```python
from build123d import *

# Parameters (mm, degrees)
SKETCH1_R           = 7.5
BOSS_EXTRUDE1_DEPTH = 40
SKETCH2_W           = 30
SKETCH2_H           = 30
SKETCH2_H_2         = 5
CUT_EXTRUDE1_DEPTH  = 162.686727154


with BuildPart() as part:
    # Sketch1 → Boss-Extrude1 (new body)
    with BuildSketch(Plane.XY):
        with BuildLine():
            Line((0, 15), (138.761496278, 15))
            ThreePointArc((138.761496278, 15), (153.761496278, 0), (138.761496278, -15))
            Line((138.761496278, -15), (0, -15))
            ThreePointArc((0, -15), (-15, 0), (0, 15))
        make_face()
        Circle(SKETCH1_R, mode=Mode.SUBTRACT)
        with Locations((138.761496278, 0)):
            Circle(SKETCH1_R, mode=Mode.SUBTRACT)
    extrude(amount=BOSS_EXTRUDE1_DEPTH)

    # Sketch2 → Cut-Extrude1 (cut, through all)
    with BuildSketch(Plane(origin=(0, 15, 0), x_dir=(1, 0, 0), z_dir=(0, 1, 0))):
        with Locations((0, -20)):
            Rectangle(SKETCH2_W, SKETCH2_H)
        with Locations((138.761496278, -2.5)):
            Rectangle(SKETCH2_W, SKETCH2_H_2)
        with Locations((138.761496278, -37.5)):
            Rectangle(SKETCH2_W, SKETCH2_H_2)
    extrude(amount=-CUT_EXTRUDE1_DEPTH, mode=Mode.SUBTRACT)


solid = part.part
```
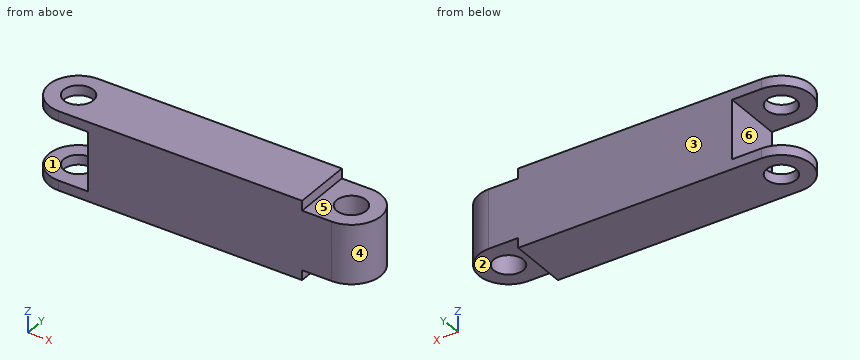
Check sheet for the modelled part. Datum: model origin and axes. Units: mm. Face numbers are marked on the shaded views. A direction names the side the tool comes from. Coordinates: 2 decimals unless noted, no trailing zeros. Write each loop counter-clockwise with the first axis right and the second up, starting at its lowest first coordinate (ties: lowest second). Pieces come first, ordered by that corner, then holes. Notation, with made-up numbers: M -37.75,17.25 L 5.25,17.25 A26 cw 5.25,44.25 Z; hole C 29.5,-31 d9. An arc over 180 degrees is marked long. Write item = value, one per line. Start each with the question number.
1. Sectioned sample at A-A (y = 0). Record the cut outline in (x, z).
2. Sectioned sample at C-C (z = 21). Record the cut outline in (x, y).
3. Tool access check on the marked faces 4, 5 and 6. Record the directions out of +Z, -Z, +X, -X, +Y, -Y that give a thin tool (end or side, any length) a straight path to the whole face; none if there is none.
4. Go/stop test with flat-tipped pins: pin 1 (10 mm diameter, centred on y = -3, z = 25.5, fed in from +X); pin 2 (9 mm diameter, centred on x = 138.5, y = 4, fed in from +Z); pin 3 (8 mm diameter, centred on y = 1, z = 15, fed in from -X); pin 4 (2.5 mm diameter, centred on y = -3, z = 3, fed in from +X). Record where each tip stops, or that it passes through.
5. Thickness scan on probe 1 along X at (y, z) = (0, 36.55); probe 2 along Y at (x, z) = (0, 2.5); probe 3 along Z at (x, y) = (3.5, -10.5). Record the ranges inside material, lowest first.
6. Sectioned sample at B-B (x = 2.5). Record the cut outline in (y, z), then the cut area to 3 significant figures.
7. Mould release check, pull along Z, two halves, no side actions. Record for the marked faces 1, 2 and 3: pulls with the +Z half, pulls with the -Z half, needs draft (parallel to the pull), parting line crosses it, or undercut.
8. Sectioned sample at D-D (y = -11). Record the cut outline in (x, z), then the cut area to 3 significant figures.
The answers:
q1.outline = M -15,0 L -7.5,0 L -7.5,5 L -15,5 Z; M -15,35 L -7.5,35 L -7.5,40 L -15,40 Z; M 7.5,0 L 123.76,0 L 123.76,5 L 131.26,5 L 131.26,35 L 123.76,35 L 123.76,40 L 7.5,40 L 7.5,35 L 15,35 L 15,5 L 7.5,5 Z; M 146.26,5 L 153.76,5 L 153.76,35 L 146.26,35 Z
q2.outline = M 15,-15 L 138.76,-15 A15 ccw 138.76,15 L 15,15 Z; hole C 138.76,0 d15
q3.face_4 = +Z, -Z, +X
q3.face_5 = +Z, +X, +Y, -Y
q3.face_6 = -X, +Y, -Y
q4.pin_1 = 153.76
q4.pin_2 = 35
q4.pin_3 = 15
q4.pin_4 = 123.76
q5.probe_1 = -15 to -7.5, 7.5 to 123.76
q5.probe_2 = -15 to -7.5, 7.5 to 15
q5.probe_3 = 0 to 5, 35 to 40
q6.outline = M -15,0 L -7.07,0 L -7.07,5 L -15,5 Z; M -15,35 L -7.07,35 L -7.07,40 L -15,40 Z; M 7.07,0 L 15,0 L 15,5 L 7.07,5 Z; M 7.07,35 L 15,35 L 15,40 L 7.07,40 Z
q6.area = 159 mm²
q7.face_1 = undercut
q7.face_2 = pulls with the -Z half
q7.face_3 = needs draft
q8.outline = M -10.2,0 L 123.76,0 L 123.76,5 L 148.96,5 L 148.96,35 L 123.76,35 L 123.76,40 L -10.2,40 L -10.2,35 L 15,35 L 15,5 L -10.2,5 Z
q8.area = 5,360 mm²
